Design review of the part built by this model. Coordinates are the model's own, in mm. A direction names the side the tool comes from. Round coordinates to 2 decimals unless told otherwise and drop trailing zeros. Loops run counter-clockwise (first coordinate to the right, second up) from the corner with the lowest first, then second, coordinate; pieces in that order, holes last. Notation, with made-up numbers: (-39.5, 28) - (12.5, 28) arc R20 ccw to (12.5, 63) - close; hole circle Ø3 at (80, -6). An arc over 180 degrees is marked (long way). Use one line per item in the form item = value. Start each with the question number.
(1) We need section B-B, the plane y = 0. Write out the cut boundary in (x, z) (1 decimal).
(2) We need section C-C, the plane z = 2.45. Give the number of separate pieces and of enclosed holes in the cut face, then the cut area to 3 significant figures.
(3) Machinability: for faces 4 (the cylindrical face through (-5.6, -12.8, 1.6)), 5 (the cylindrical face through (39.739, 68.705, 1.565)), which of the approach directions +Z, -Z, +X, -X, +Y, -Y give a long, thin tool a straight path to every point of the face, cutting with its end or side? Answer none if there is none.
(4) For pin 1 (1.6 mm diameter, centred on x = 27.5, z = 2, fed in from +Y); pin 2 (7.5 mm diameter, centred on x = 0, y = 137.668, fed in from -Z), all flat-tipped, find the tip position at first contact; note any pin that passes through.
(5) We need section A-A, the plane y = 24. Write out the cut boundary in (x, z) (3 decimals), then the cut area to 3 significant figures.
(6) The part is to be moulded in two halves that separate along Y. For faces 1 (the cylindrical face through (50.735, 61.254, 1.565)), 2 (the cylindrical face through (12.78, 79.77, 1.61)), 3 (the flat face through (19, 61, 3.175)), say which applies: released by +Y, released by -Y, zero draft, split by the parting line, or undercut.
(7) Wall thickness on probe 1 along Y at (x, z) = (34.5, 2.3); probe 2 along Y at (x, z) = (-2.5, 2.65); probe 3 along Y at (x, z) = (31.5, 2.2): over which ranges is each line inside the solid? List them lowest first. Write a range as [from, to].
from build123d import *

# Parameters (mm, degrees)
SKETCH1_R           = 7.8105
SKETCH1_R_2         = 3.3655
SKETCH1_R_3         = 4.191
BOSS_EXTRUDE1_DEPTH = 3.175
CUT_EXTRUDE1_DEPTH  = 6.35
FILLET1_R           = 2.54
FILLET5_R           = 7.62


with BuildPart() as part:
    # Sketch1 → Boss-Extrude1 (new body)
    with BuildSketch(Plane.XY):
        with BuildLine():
            Line((8.98309661, 142.414532976), (49.565953559, 65.609056962))
            ThreePointArc((49.565953559, 65.609056962), (50.742856949, 60.862523985), (49.565953559, 56.115991009))
            Line((49.565953559, 56.115991009), (8.177790267, -11.326281223))
            ThreePointArc((8.177790267, -11.326281223), (-6.360706327, -12.437938536), (-13.97, 0))
            ThreePointArc((-13.97, 0), (7.886144716, 68.281846548), (-10.16, 137.668))
            ThreePointArc((-10.16, 137.668), (-2.445131739, 147.529385845), (8.98309661, 142.414532976))
        make_face()
        Circle(SKETCH1_R, mode=Mode.SUBTRACT)
        with Locations((40.582856949, 60.862523985)):
            Circle(SKETCH1_R_2, mode=Mode.SUBTRACT)
        with Locations((0, 137.668)):
            Circle(SKETCH1_R_3, mode=Mode.SUBTRACT)
    extrude(amount=BOSS_EXTRUDE1_DEPTH)

    # Sketch2 → Cut-Extrude1 (cut)
    with BuildSketch(Plane.XY.offset(3.175)):
        with BuildLine():
            ThreePointArc((-1.687172275, 10.855167431), (6.949528794, 8.507952738), (10.973487677, 0.513593659))
            Line((10.973487677, 0.513593659), (36.90141673, 42.763317023))
            Line((36.90141673, 42.763317023), (-1.687172275, 10.855167431))
        make_face()
        with BuildLine():
            ThreePointArc((12.283170574, 57.862523985), (9.009504683, 39.343064628), (3.172468256, 21.465249632))
            Line((3.172468256, 21.465249632), (44.364286203, 55.525958325))
            ThreePointArc((44.364286203, 55.525958325), (39.035089517, 54.507796908), (34.770960507, 57.862523985))
            Line((34.770960507, 57.862523985), (12.283170574, 57.862523985))
        make_face()
        with BuildLine():
            Line((5.700051608, 115.487969959), (37.341521976, 80.589180404))
            Line((37.341521976, 80.589180404), (7.358422957, 137.33398266))
            ThreePointArc((7.358422957, 137.33398266), (4.930965477, 132.195931336), (-0.431201431, 130.314631974))
            ThreePointArc((-0.431201431, 130.314631974), (2.856784408, 122.993252968), (5.700051608, 115.487969959))
        make_face()
        with BuildLine():
            ThreePointArc((34.770960507, 63.862523985), (38.185315424, 66.94774665), (42.786522834, 67.020607852))
            Line((42.786522834, 67.020607852), (9.033823823, 104.247965684))
            ThreePointArc((9.033823823, 104.247965684), (12.444109183, 84.197859008), (12.777235899, 63.862523985))
            Line((12.777235899, 63.862523985), (34.770960507, 63.862523985))
        make_face()
    extrude(amount=-CUT_EXTRUDE1_DEPTH, mode=Mode.SUBTRACT)

    # Fillet1
    fillet1_edges = [part.edges().sort_by_distance(p)[0] for p in [
        (44.364286203, 55.525958325, 1.5875),
        (3.172468256, 21.465249632, 1.5875),
        (42.786522834, 67.020607852, 1.5875),
        (34.770960507, 63.862523985, 1.5875),
        (9.033823823, 104.247965684, 1.5875),
        (-0.431201431, 130.314631974, 1.5875),
        (7.358422957, 137.33398266, 1.5875),
        (37.341521976, 80.589180404, 1.5875),
        (5.700051608, 115.487969959, 1.5875),
        (10.973487677, 0.513593659, 1.5875),
        (-1.687172275, 10.855167431, 1.5875),
        (36.90141673, 42.763317023, 1.5875),
    ]]
    fillet(fillet1_edges, radius=FILLET1_R)

    # Fillet5
    # the kernel refuses this fillet: 7.62 mm, written as the material it takes off along each edge
    with BuildSketch(Plane(origin=(49.565953559, 56.115991009, -1.635210381), x_dir=(0.4384758636480836, 0.8987429649227121, 0), z_dir=(0, 0, 1))) as fillet5_piece_1:
        with BuildLine():
            CenterArc((0.408802595, 7.616051271), FILLET5_R, 264.46995043, 7.374672414)
            Line((-0.325519955, 0.031516322), (0, 0))
            ThreePointArc((0, 0), (0.327042076, -0.005264972), (0.654084152, 0))
        make_face()
    extrude(amount=6.445420761, mode=Mode.SUBTRACT)
    with BuildSketch(Plane(origin=(8.177790267, -11.326281223, -6.821790927), x_dir=(-0.8640520418582298, -0.5034024920087542, 0), z_dir=(0, 0, 1))) as fillet5_piece_2:
        with BuildLine():
            CenterArc((1.984520997, -7.583572591), FILLET5_R, 84.39536353, 33.842547752)
            Line((-1.620758554, -0.870424346), (0, 0))
            ThreePointArc((0, 0), (1.364358185, 0.066783583), (2.728716371, 0))
        make_face()
    extrude(amount=16.818581854, mode=Mode.SUBTRACT)
    with BuildSketch(Plane(origin=(-13.97, 0, -10.324988133), x_dir=(0.5491862360699723, 0.8356999928869789, 0), z_dir=(0, 0, 1))) as fillet5_piece_3:
        with BuildLine():
            CenterArc((2.785592727, -7.619579496), FILLET5_R, 90.601931521, 49.710102388)
            ThreePointArc((-3.078254062, -2.753400211), (-1.641438538, -1.262317601), (0, 0))
            ThreePointArc((0, 0), (1.352770433, -0.007105957), (2.705540865, 0))
        make_face()
    extrude(amount=23.824976265, mode=Mode.SUBTRACT)
    with BuildSketch(Plane(origin=(-10.16, 137.668, -14.214457568), x_dir=(0.2798121568434471, 0.96005476764746, 0), z_dir=(0, 0, 1))) as fillet5_piece_4:
        with BuildLine():
            CenterArc((3.553614392, -7.315617329), FILLET5_R, 73.751006034, 62.011444153)
            ThreePointArc((-1.90576169, -1.999640205), (-0.947518647, -1.004930558), (0, 0))
            ThreePointArc((0, 0), (2.842891514, 0.405843561), (5.685783027, 0))
        make_face()
    extrude(amount=31.603915135, mode=Mode.SUBTRACT)


solid = part.part
Data:
q1.outline = (-13.5, 0) - (-7.8, 0) - (-7.8, 3.2) - (-13.5, 3.2) - close; (7.8, 0) - (15.1, 0) - (15.1, 3.2) - (7.8, 3.2) - close
q2.separate_pieces = 1
q2.enclosed_holes = 7
q2.area = 2,640 mm^2
q3.face_4 = +Z, -Z, -Y
q3.face_5 = +Z, -Z
q4.pin_1 = 108.88
q4.pin_2 = through
q5.outline = (-1.283, 0) - (14.21, 0) - (14.21, 3.175) - (-1.283, 3.175) - close; (25.387, 0) - (29.857, 0) - (29.857, 3.175) - (25.387, 3.175) - close
q5.area = 63.4 mm^2
q6.face_1 = split by the parting line
q6.face_2 = undercut
q6.face_3 = zero draft
q7.probe_1 = [31.57, 47.37], [57.86, 64.12], [76.16, 94.12]
q7.probe_2 = [-13.74, -7.4], [7.4, 21.06], [122.62, 134.3], [141.03, 147.52]
q7.probe_3 = [26.68, 44.89], [57.86, 63.86], [79.47, 99.8]
